from build123d import *

# Parameters (mm, degrees)
SKETCH1_R           = 1.3335
SKETCH1_R_2         = 1.143
BOSS_EXTRUDE1_DEPTH = 3.175


with BuildPart() as part:
    # Sketch1 → Boss-Extrude1 (new body)
    with BuildSketch(Plane.XY):
        Polygon((0, 0), (4.613655526, 5.08), (24.933655526, 5.08), (24.933655526, 9.671782949), (29.21, 9.671782949), (29.21, 21.59), (38.1, 21.59), (38.1, 0), (15.700557681, 0), (15.700557681, 1.020592656), (14.773655526, 0), align=None)
        with Locations((29.033993158, 3.299509856)):
            Circle(SKETCH1_R, mode=Mode.SUBTRACT)
        with Locations((35.383993158, 3.299509856)):
            Circle(SKETCH1_R, mode=Mode.SUBTRACT)
        with Locations((34.29, 16.51)):
            Circle(SKETCH1_R_2, mode=Mode.SUBTRACT)
    extrude(amount=BOSS_EXTRUDE1_DEPTH)


solid = part.part
Here's how the part is built. I have some questions about the finished solid (model axes, mm). A direction names the side the tool comes from. Round coordinates to 2 decimals unless told otherwise and drop trailing zeros. Loops run counter-clockwise (first coordinate to the right, second up) from the corner with the lowest first, then second, coordinate; pieces in that order, holes last. Notation, with made-up numbers: (89, -5.75) - (147, -5.75) arc R32 ccw to (147, 33.25) - close; hole circle Ø9 at (-6, 76.5). An arc over 180 degrees is marked (long way). One line per question, with ' | ' between items. Start each with the question number.
Q1. We'd pull the mould along X, two halves only. Please class faces 3 (the flat face through (24.934, 7, 2)), 4 (the flat face through (15, 5.08, 2)), 5 (the cylindrical face through (27.7, 3.36, 1.57)): +X half, -X half, draft (parallel to the pull), parting line (faces both ways), or undercut.
Q2. Please list where these lines run through material, in increasing order: line 1 (Y direction, x = 34.29, z = 2); line 2 (Y direction, x = 35, z = 2.3); line 3 (X direction, y = 2.5, z = 2.85). Write a range as [from, to].
Q3. I want a section at B-B (y = 3.75). Write out the boundary of the cut face in (x, z) (3 decimals), then the cut area to 3 significant figures.
Q4. I want a section at D-D (x = 17.5). Write out the boundary of the cut face in (y, z) (3 decimals).
Q5. For faces 1 (the flat face through (28, 9, 0)), 2 (the flat face through (29.21, 16, 2)), which set-ups out of +Z, -Z, +X, -X, +Y, -Y let a thin tool reach every point of the face, with its end or its side?
Q6. I want a section at A-A (y = 16.51). Write out the boundary of the cut face in (x, z) (3 decimals), then the cut area to 3 significant figures.
Q7. Will these pins go through, and if not, where does the flat tip stop? pin 1 (6 mm diameter, centred on x = 5.5, y = 10, fed in from -Z); pin 2 (8 mm diameter, centred on x = 15.5, y = 7, fed in from -Z).
Q8. I want a section at C-C (z = 2.6). Write out the boundary of the cut face in (x, y), then the cut area to 3 significant figures.
Response values:
1) face 3: -X half | face 4: draft | face 5: undercut
2) line 1: y = [0, 2.54], [4.06, 15.37], [17.65, 21.59] | line 2: y = [0, 2.02], [4.58, 15.61], [17.41, 21.59] | line 3: x = [2.27, 27.97], [30.1, 34.32], [36.45, 38.1]
3) outline: (3.406, 0) - (27.779, 0) - (27.779, 3.175) - (3.406, 3.175) - close; (30.289, 0) - (34.129, 0) - (34.129, 3.175) - (30.289, 3.175) - close; (36.639, 0) - (38.1, 0) - (38.1, 3.175) - (36.639, 3.175) - close | area: 94.2 mm²
4) outline: (0, 0) - (5.08, 0) - (5.08, 3.175) - (0, 3.175) - close
5) face 1: -Z, +X, -X, +Y, -Y | face 2: +Z, -Z, -X, +Y
6) outline: (29.21, 0) - (33.147, 0) - (33.147, 3.175) - (29.21, 3.175) - close; (35.433, 0) - (38.1, 0) - (38.1, 3.175) - (35.433, 3.175) - close | area: 21.0 mm²
7) pin 1: passes through | pin 2: stops at z = 0
8) outline: (0, 0) - (14.77, 0) - (15.7, 1.02) - (15.7, 0) - (38.1, 0) - (38.1, 21.59) - (29.21, 21.59) - (29.21, 9.67) - (24.93, 9.67) - (24.93, 5.08) - (4.61, 5.08) - close; hole circle Ø2.67 at (29.03, 3.3); hole circle Ø2.29 at (34.29, 16.51); hole circle Ø2.67 at (35.38, 3.3) | area: 332 mm²
